Read the model definition and answer for the solid it produces. Units are mm, in the model's axes. Face numbers are marked on the shaded views. A direction names the side the tool comes from. Give positions to 0.01 mm unless a question says otherwise; leave off trailing zeros. Order: outer loops, then holes, each group sorted by start corner. A loop starts at its lowest first (then second) coordinate and runs counter-clockwise, first axis right, second up. Notation, with made-up numbers: (6, -10.5) - (61, -10.5) arc R4 ccw to (61, -5.5) - close; hole circle Ø6 at (87, 2). An arc over 180 degrees is marked (long way). Write item = value, one per line.
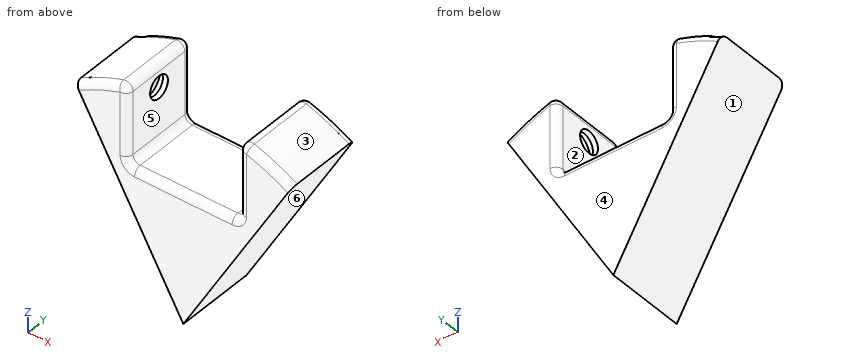
```python
from build123d import *

# Parameters (mm, degrees)
BOSS_EXTRUDE1_DEPTH = 28
CUT_EXTRUDE1_DEPTH  = 90.677477663
SKETCH5_R           = 6.35
CUT_EXTRUDE2_DEPTH  = 4.572
SKETCH8_R           = 6.35
SKETCH8_R_2         = 3.937
BOSS_EXTRUDE4_DEPTH = 1.778
FILLET1_R           = 2.54


with BuildPart() as part:
    # Sketch2 → Boss-Extrude1 (new body)
    with BuildSketch(Plane(origin=(0, 0, 0), x_dir=(1, 0, 0), z_dir=(0, 1, 0))):
        with BuildLine():
            Line((-38.1, -65.991135768), (0, 0))
            Line((0, 0), (0, -76.2))
            ThreePointArc((0, -76.2), (-19.722011237, -73.603547963), (-38.1, -65.991135768))
        make_face()
    boss_extrude1 = extrude(amount=BOSS_EXTRUDE1_DEPTH)

    # Sketch4 → Cut-Extrude1 (cut, symmetric)
    with BuildSketch(Plane(origin=(0, 28, 0), x_dir=(1, 0, 0), z_dir=(0, 1, 0))):
        Polygon((-19.722011237, -73.603547963), (-19.722011237, -45.603553163), (19.722011237, -45.603553163), (19.722011237, -73.603547963), (19.722011237, -89.083413221), (-19.722011237, -89.083413221), align=None)
    cut_extrude1 = extrude(amount=CUT_EXTRUDE1_DEPTH, both=True, mode=Mode.SUBTRACT)

    # Sketch5 → Cut-Extrude2 (cut)
    with BuildSketch(Plane(origin=(-19.722011237, 0, 0), x_dir=(0, 0, -1), z_dir=(1, 0, 0))):
        with Locations((-64.683550563, 14)):
            Circle(SKETCH5_R)
    cut_extrude2 = extrude(amount=-CUT_EXTRUDE2_DEPTH, mode=Mode.SUBTRACT)

    # Sketch8 → Boss-Extrude4 (add)
    with BuildSketch(Plane(origin=(-19.722011237, 0, 0), x_dir=(0, 0, -1), z_dir=(1, 0, 0))):
        with Locations((-64.683550563, 14)):
            Circle(SKETCH8_R)
        with Locations((-64.683550563, 14)):
            Circle(SKETCH8_R_2, mode=Mode.SUBTRACT)
    boss_extrude4 = extrude(amount=-BOSS_EXTRUDE4_DEPTH)

    # Mirror1: Boss-Extrude1, Cut-Extrude1, Cut-Extrude2, Boss-Extrude4 across plane
    add(boss_extrude1.mirror(Plane(origin=(0, 28, 0), x_dir=(0, 0, 1), z_dir=(-1, 0, 0))))
    add(cut_extrude1.mirror(Plane(origin=(0, 28, 0), x_dir=(0, 0, 1), z_dir=(-1, 0, 0))), mode=Mode.SUBTRACT)
    add(cut_extrude2.mirror(Plane(origin=(0, 28, 0), x_dir=(0, 0, 1), z_dir=(-1, 0, 0))), mode=Mode.SUBTRACT)
    add(boss_extrude4.mirror(Plane(origin=(0, 28, 0), x_dir=(0, 0, 1), z_dir=(-1, 0, 0))))

    # Fillet1
    fillet1_edges = [part.edges().sort_by_distance(p)[0] for p in [
        (0, 0, 45.603553163),
        (-29.160477546, 28, 70.399620377),
        (-19.722011237, 0, 59.603550563),
        (-19.722011237, 14, 73.603547963),
        (-19.722011237, 28, 59.603550563),
        (0, 28, 45.603553163),
        (-19.722011237, 14, 45.603553163),
        (-29.160477546, 0, 70.399620377),
        (29.160477546, 28, 70.399620377),
        (29.160477546, 0, 70.399620377),
        (19.722011237, 0, 59.603550563),
        (19.722011237, 14, 73.603547963),
        (19.722011237, 28, 59.603550563),
        (19.722011237, 14, 45.603553163),
    ]]
    fillet(fillet1_edges, radius=FILLET1_R)


solid = part.part
```
1. Determine the mould class of the marked faces 1, 2, 3 and 4 for opening direction X: +X half, -X half, draft (parallel to the pull), parting line (faces both ways), or undercut.
Recorded:
face_1 = -X half
face_2 = undercut
face_3 = +X half
face_4 = draft
2. For the marked faces 5 and 6, determine the directions among +Z, -Z, +X, -X, +Y, -Y from which every point of the face is accessible in a straight line to the end or side of a thin tool.
Recorded:
face_5 = +Z, +Y, -Y
face_6 = -Z, +X, +Y, -Y
3. Section C-C (y = 14) is taken. Determine the outline of the cut face in (x, z).
Recorded:
outline = (-38.1, 65.99) - (0, 0) - (38.1, 65.99) arc R76.2 ccw to (23.03, 72.64) arc R2.54 ccw to (19.72, 70.22) - (19.72, 68.62) - (21.5, 68.62) - (21.5, 71.03) - (24.29, 71.03) - (24.29, 58.33) - (21.5, 58.33) - (21.5, 60.75) - (19.72, 60.75) - (19.72, 48.14) arc R2.54 cw to (17.18, 45.6) - (-17.18, 45.6) arc R2.54 cw to (-19.72, 48.14) - (-19.72, 60.75) - (-21.5, 60.75) - (-21.5, 58.33) - (-24.29, 58.33) - (-24.29, 71.03) - (-21.5, 71.03) - (-21.5, 68.62) - (-19.72, 68.62) - (-19.72, 70.22) arc R2.54 ccw to (-23.03, 72.64) arc R76.2 ccw to start
4. Section D-D (z = 39) is taken. Determine the outline of the cut face in (x, y), and give its area (3 significant figures).
Recorded:
outline = (-22.52, 0) - (22.52, 0) - (22.52, 28) - (-22.52, 28) - close
area = 1,260 mm^2
5. Section A-A (y = 3.5) is taken. Determine the outline of the cut face in (x, z).
Recorded:
outline = (-38.1, 65.99) - (0, 0) - (38.1, 65.99) arc R76.2 ccw to (23.03, 72.64) arc R2.54 ccw to (19.72, 70.22) - (19.72, 48.14) arc R2.54 cw to (17.18, 45.6) - (-17.18, 45.6) arc R2.54 cw to (-19.72, 48.14) - (-19.72, 70.22) arc R2.54 ccw to (-23.03, 72.64) arc R76.2 ccw to start
6. Flat-ended cylindrical pins translate along their axes: pin 1 (1 mm diameter, centred on y = 12.5, z = 45.5, fed in from -X); pin 2 (10 mm diameter, centred on y = 14, z = 64.68, fed in from +X); pin 3 (11 mm diameter, centred on y = 10, z = 59.5, fed in from +X). Find the tip coordinate at first contact, or state that the pin passes through.
Recorded:
pin_1 = -26.56
pin_2 = 38.1
pin_3 = 37.53
7. Section B-B (z = 62.5) is taken. Determine the outline of the cut face in (x, y).
Recorded:
outline = (-36.08, 0) - (-22.26, 0) arc R2.54 ccw to (-19.72, 2.54) - (-19.72, 10.72) - (-21.5, 10.72) - (-21.5, 8.04) - (-24.29, 8.04) - (-24.29, 19.96) - (-21.5, 19.96) - (-21.5, 17.28) - (-19.72, 17.28) - (-19.72, 25.46) arc R2.54 ccw to (-22.26, 28) - (-36.08, 28) - close; (19.72, 2.54) arc R2.54 ccw to (22.26, 0) - (36.08, 0) - (36.08, 28) - (22.26, 28) arc R2.54 ccw to (19.72, 25.46) - (19.72, 17.28) - (21.5, 17.28) - (21.5, 19.96) - (24.29, 19.96) - (24.29, 8.04) - (21.5, 8.04) - (21.5, 10.72) - (19.72, 10.72) - close
8. Straight lines are drawn through the part: L1, parallel to X at y = 5.75, z = 63.5; L2, parallel to X at y = 20.75, z = 64; L3, parallel to X at y = 27, z = 4.5. For each, find the intervals that lie inside material, in ascending order. Write a range as [from, to].
Recorded:
L1 = [-36.66, -19.72], [19.72, 36.66]
L2 = [-36.95, -19.72], [19.72, 36.95]
L3 = [-2.6, 2.6]
